from build123d import *

# Parameters (mm, degrees)
F0_W     = 75
F0_H     = 45
F1_DEPTH = 7.5
F2_T     = -2.5
F3_W     = 75
F3_H     = 45
F4_DEPTH = 2.5
F5_R     = 6.5
F6_DEPTH = 37


with BuildPart() as f1:
    # F0 (on Top) → F1 (new body, symmetric)
    with BuildSketch(Plane.XY):
        Rectangle(F0_W, F0_H)
    extrude(amount=F1_DEPTH, both=True)

    # F2
    f2_openings = [f1.faces().sort_by_distance(p)[0] for p in [
        (0, 0, 7.5),
    ]]
    offset(amount=F2_T, openings=f2_openings)

    # F3 (on face) → F4 (join)
    with BuildSketch(Plane.XY.offset(7.5)):
        Rectangle(F3_W, F3_H)
    extrude(amount=F4_DEPTH)

    # F5 (on Right) → F6 (join, symmetric)
    with BuildSketch(Plane.YZ):
        with Locations((0, 1.25)):
            Circle(F5_R)
    extrude(amount=F6_DEPTH, both=True)


solid = f1.part
Geometry: final body of the model. Coordinates: model frame, mm. A direction names the side the tool comes from. Coordinates: 2 decimals unless noted, no trailing zeros. Loops run counter-clockwise (first coordinate to the right, second up) from the corner with the lowest first, then second, coordinate; pieces in that order, holes last. Notation, with made-up numbers: (8, -29) - (27, -29) arc R19 cw to (27, 8) - close; hole circle Ø7 at (33.25, -36.5). An arc over 180 degrees is marked (long way). Put each result on its own line as item: value. Start each with the question number.
Q1. Line query: line 1 (Y direction, x = 13.5, z = 1); line 2 (Z direction, x = -24, y = -11.5); line 3 (X direction, y = 8, z = -3). Output: solid intervals per line, ascending.
Q2. Pull-direction query (Y, two-part tool) for faces 3 (the flat face through (-1, 22.5, 1)), 4 (the flat face through (0, -20, 1)), 5 (the flat face through (-37.5, 0, 1)), 6 (the cylindrical face through (0.5, 6.5, 1.1)); classes: released by +Y, released by -Y, zero draft, split by the parting line, or undercut.
Q3. Set-up query: faces 1 (the flat face through (-1, -22.5, 1)), 2 (the flat face through (0, -11, -5)). Return all of +Z, -Z, +X, -X, +Y, -Y with unobstructed straight access to the full face (end or side cutting, diameter ignored); none if empty.
Q4. Cut plane C-C, the plane x = 3. Return loops of the section in (y, z).
Q5. Cut plane A-A, the plane z = 3. Return loops of the section in (x, y).
Q6. Cut plane B-B, the plane y = 13.5. Return loops of the section in (x, z), and give its area (4 significant figures).
Filled sheet:
1. line 1: -22.5 to -20, -6.5 to 6.5, 20 to 22.5
1. line 2: -7.5 to -5, 7.5 to 10
1. line 3: -37.5 to -35, 35 to 37.5
2. face 3: released by +Y
2. face 4: undercut
2. face 5: zero draft
2. face 6: undercut
3. face 1: +Z, -Z, +X, -X, -Y
3. face 2: none
4. outline: (-22.5, -7.5) - (22.5, -7.5) - (22.5, 10) - (-22.5, 10) - close; hole (-20, -5) - (-1.79, -5) arc R6.5 cw to (-1.79, 7.5) - (-20, 7.5) - close; hole (1.79, -5) - (20, -5) - (20, 7.5) - (1.79, 7.5) arc R6.5 cw to start
5. outline: (-37.5, -22.5) - (37.5, -22.5) - (37.5, 22.5) - (-37.5, 22.5) - close; hole (-35, -20) - (35, -20) - (35, -6.26) - (-35, -6.26) - close; hole (-35, 6.26) - (35, 6.26) - (35, 20) - (-35, 20) - close
6. outline: (-37.5, -7.5) - (37.5, -7.5) - (37.5, 10) - (-37.5, 10) - close; hole (-35, -5) - (35, -5) - (35, 7.5) - (-35, 7.5) - close
6. area: 437.5 mm²
